The model under review builds one solid part; all positions refer to its coordinate system, in mm. A direction names the side the tool comes from. Round coordinates to 2 decimals unless told otherwise and drop trailing zeros. Loops run counter-clockwise (first coordinate to the right, second up) from the corner with the lowest first, then second, coordinate; pieces in that order, holes last. Notation, with made-up numbers: M -38,73.25 L -32,73.25 A33 cw -32,106.25 Z; hole C 86,-20.75 d11. An arc over 180 degrees is marked long. Return JSON: item names as keys, results as strings. Group by question number.
Q1. Consider section C-C (z = -1.5). State the section outline as (x, y) points (3 decimals), and give its area (3 significant figures).
Q2. Consider section A-A (z = -6.35). State the section outline as (x, y) points (3 decimals), and give its area (3 significant figures).
Q3. To check wall thickness, follow line 1 along X through (y, z) = (8, -5.25) (3 decimals); line 2 along Y through (x, z) = (2.25, -6.35); line 3 along Y through (x, z) = (19, -6.5) (3 decimals). State the ranges of each line that lie inside material, in increasing order.
Q4. Consider section D-D (y = 16.5). State the section outline as (x, z) points (3 decimals).
Q5. Draft analysis for pull direction X (two halves, no side actions). For faces 3 (the face through (30, 19.05, -6)), 4 (the face through (16, 3.175, -6)), 5 (the face through (0, 10, -6)), 6 (the face through (31.75, 10, -6)), state which applies: pulls with the +X half, pulls with the -X half, needs draft (parallel to the pull), parting line crosses it, or undercut.
Q6. For faces 1 (the face through (3.175, 11, -6)), 2 (the face through (2, 19.05, -6)), list the 3-axis set-ups (+Z, -Z, +X, -X, +Y, -Y) from which the entire face can be reached by the end or side of a thin tool; tool diameter is ignored.
Q7. Consider section B-B (y = 9). State the section outline as (x, z) points (3 decimals).
Q8. Clearance check with flat-ended pins moving along their axes: pin 1 Ø1.5 at (x, z) = (20, -2.5) entering from -Y; pin 2 Ø8 at (x, y) = (23.5, 13) entering from +Z; pin 3 Ø2 at (x, z) = (25.5, -7.5) entering from +Y (3 decimals). State where each tip first meets the part, or that it passes through.
from build123d import *

# Parameters (mm, degrees)
SKETCH1_W                      = 12.7
SKETCH1_H                      = 19.05
BOSS_EXTRUDE1_DEPTH            = 31.75
CUT_EXTRUDE1_REACH             = 41.144
SKETCH2_W                      = 25.4
SKETCH2_H                      = 15.875
F_3_16_0_1875_DIAMETER_HOLE1_D = 4.7625


with BuildPart() as part:
    # Sketch1 → Boss-Extrude1 (new body)
    with BuildSketch(Plane(origin=(0, 0, 0), x_dir=(0, 0, -1), z_dir=(1, 0, 0))):
        with Locations((6.35, 9.525)):
            Rectangle(SKETCH1_W, SKETCH1_H)
    extrude(amount=BOSS_EXTRUDE1_DEPTH)

    # Sketch2 → Cut-Extrude1 (cut, up to next)
    with BuildSketch(Plane.XY, mode=Mode.PRIVATE) as cut_extrude1_sk1:
        with Locations((15.875, 11.1125)):
            Rectangle(SKETCH2_W, SKETCH2_H)
    cut_extrude1_tool1 = extrude(cut_extrude1_sk1.sketch, amount=-CUT_EXTRUDE1_REACH, mode=Mode.PRIVATE) & part.part
    add(cut_extrude1_tool1.solids().sort_by_distance((15.875, 11.1125, 0))[0], mode=Mode.SUBTRACT)

    # 3/16 (0.1875) Diameter Hole1 (through all)
    with Locations(Plane(origin=(31.75, 0, 0), x_dir=(0, 0, -1), z_dir=(1, 0, 0))):
        with Locations((6.35, 15.875)):
            Hole(F_3_16_0_1875_DIAMETER_HOLE1_D / 2)


solid = part.part
Values:
{
 "1": {"outline": "M 0,0 L 31.75,0 L 31.75,19.05 L 28.575,19.05 L 28.575,3.175 L 3.175,3.175 L 3.175,19.05 L 0,19.05 Z", "area": "202 mm2"},
 "2": {"outline": "M 0,0 L 31.75,0 L 31.75,13.494 L 28.575,13.494 L 28.575,3.175 L 3.175,3.175 L 3.175,13.494 L 0,13.494 Z; M 0,18.256 L 3.175,18.256 L 3.175,19.05 L 0,19.05 Z; M 28.575,18.256 L 31.75,18.256 L 31.75,19.05 L 28.575,19.05 Z", "area": "171 mm2"},
 "3": {"line 1": "x = 0 to 3.175, 28.575 to 31.75", "line 2": "y = 0 to 13.49, 18.26 to 19.05", "line 3": "y = 0 to 3.175"},
 "4": {"outline": "M 0,-12.7 L 3.175,-12.7 L 3.175,-8.648 L 0,-8.648 Z; M 0,-4.052 L 3.175,-4.052 L 3.175,0 L 0,0 Z; M 28.575,-12.7 L 31.75,-12.7 L 31.75,-8.648 L 28.575,-8.648 Z; M 28.575,-4.052 L 31.75,-4.052 L 31.75,0 L 28.575,0 Z"},
 "5": {"face 3": "needs draft", "face 4": "undercut", "face 5": "pulls with the -X half", "face 6": "pulls with the +X half"},
 "6": {"face 1": "+Z, -Z, +Y", "face 2": "+Z, -Z, +X, -X, +Y"},
 "7": {"outline": "M 0,-12.7 L 3.175,-12.7 L 3.175,0 L 0,0 Z; M 28.575,-12.7 L 31.75,-12.7 L 31.75,0 L 28.575,0 Z"},
 "8": {"pin 1": "stops at y = 0", "pin 2": "passes through", "pin 3": "stops at y = 3.175"}
}
